Could you check a few things on this drawing? It's one solid part, dimensions in mm from its lowest x, y, z. A direction names the side the tool comes from. Coordinates: 2 decimals unless noted, no trailing zeros. Write each loop counter-clockwise with the first axis right and the second up, starting at its lowest first coordinate (ties: lowest second). Pieces come first, ordered by that corner, then holes. Notation, with made-up numbers: (-33, -39) - (-25, -39) arc R29 ccw to (-25, -12) - close; hole circle Ø4 at (12.5, 88). An arc over 180 degrees is marked (long way). Use one line per item in the form item = value. Start each with the question number.
(1) For pin 1 Ø10 at (y, z) = (24.5, 6) entering from +X; pin 2 Ø3 at (x, z) = (43, 12.5) entering from -Y, each with a flat end and sliding along its axis, tell me the tip position at first contact or that it passes through.
(2) If we section it at A-A on z = 9: Please give me the cut outline in (x, y) (1 decimal).
(3) On a 3-axis mill with a long thin cutter (end or side, diameter ignored), from which of +Z, -Z, +X, -X, +Y, -Y can I reach the whole of each face in a straight line? I mean the marked faces 1, 2, 3, 4 and 5. Say none if no direction works.
(4) If I drill on probe 1 along Z at (x, y) = (45, 17.25) (1 decimal); probe 2 along X at (y, z) = (8.75, 10) (1 decimal); probe 3 along Y at (x, z) = (100.5, 6), over which ranges is the centre line in solid material (lowest first)? Write a range as from..to.
(5) If we section it at C-C on y = 7: Please give me the cut outline in (x, z) (1 decimal), then the cut area to 3 significant figures.
(6) If we section it at B-B on y = 23: Please give me the cut outline in (x, z) (1 decimal).
(7) If we section it at D-D on x = 80: Please give me the cut outline in (y, z) (1 decimal).
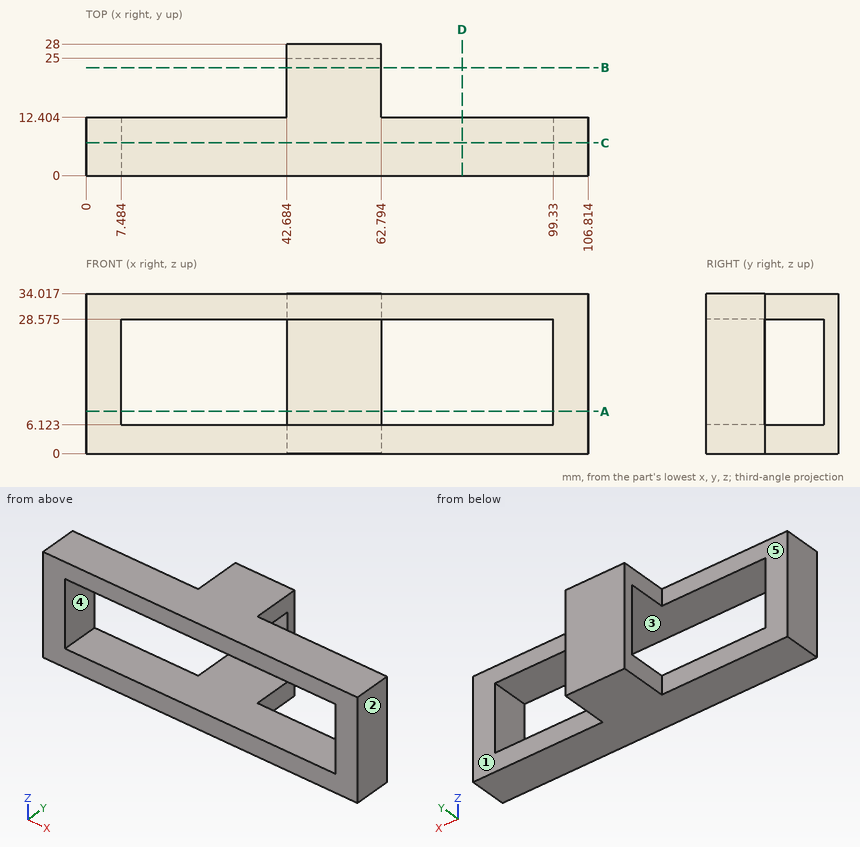
Reported:
q1.pin_1 = 62.79
q1.pin_2 = 25
q2.outline = (0, 0) - (7.5, 0) - (7.5, 12.4) - (0, 12.4) - close; (42.7, 25) - (62.8, 25) - (62.8, 28) - (42.7, 28) - close; (99.3, 0) - (106.8, 0) - (106.8, 12.4) - (99.3, 12.4) - close
q3.face_1 = +Z, -Z, +X, +Y
q3.face_2 = +Z, -Z, +X, +Y, -Y
q3.face_3 = -Y
q3.face_4 = +Y, -Y
q3.face_5 = +Z, -Z, -X, +Y
q4.probe_1 = 0..6.1, 28.6..34
q4.probe_2 = 0..7.5, 99.3..106.8
q4.probe_3 = 0..12.4
q5.outline = (0, 0) - (106.8, 0) - (106.8, 34) - (0, 34) - close; hole (7.5, 6.1) - (99.3, 6.1) - (99.3, 28.6) - (7.5, 28.6) - close
q5.area = 1,570 mm2
q6.outline = (42.7, 0) - (62.8, 0) - (62.8, 6.1) - (42.7, 6.1) - close; (42.7, 28.6) - (62.8, 28.6) - (62.8, 34) - (42.7, 34) - close
q7.outline = (0, 0) - (12.4, 0) - (12.4, 6.1) - (0, 6.1) - close; (0, 28.6) - (12.4, 28.6) - (12.4, 34) - (0, 34) - close
